Study the drawing (mm; zero at the part's minimum x, y, z) and answer. A direction names the side the tool comes from. Round coordinates to 2 decimals unless told otherwise and drop trailing zeros. Write each loop counter-clockwise with the first axis right and the second up, starting at its lowest first coordinate (ties: lowest second). Pieces come first, ordered by that corner, then holes. Notation, with made-up numbers: (59, -11.5) - (65, -11.5) arc R27 ccw to (65, 25.5) - close; hole circle Ø6 at (80, 0). An arc over 180 degrees is marked (long way). Return JSON: item names as keys, results as strings. Group by question number.
(1) Section A-A, the plane z = 55.5 is taken. Write down the section's boundary in (x, y), then the cut area to 3 significant figures.
(2) Which of the six approach directions +Z, -Z, +X, -X, +Y, -Y give full straight-line access (tool end or side, diameter ignored) to the marked faces 1 and 2?
(3) Section B-B, the plane x = 34 is taken. Write down the section's boundary in (y, z), then the cut area to 3 significant figures.
(4) Find the intervals of material crossed by line 1 along Y through (x, z) = (91, 95); line 2 along Z through (x, y) = (115, 172), in increasing order. Write a range as [from, to].
(5) This flat-tipped pin is pushed along its axis until it touches: pin 1 (4 mm diameter, centred on x = 173.5, y = 196, fed in from +Z). Where does it stop, or does it pass through?
(6) Determine the mould class of the marked faces 3, 4 and 5 for opening direction X: +X half, -X half, draft (parallel to the pull), parting line (faces both ways), or undercut.
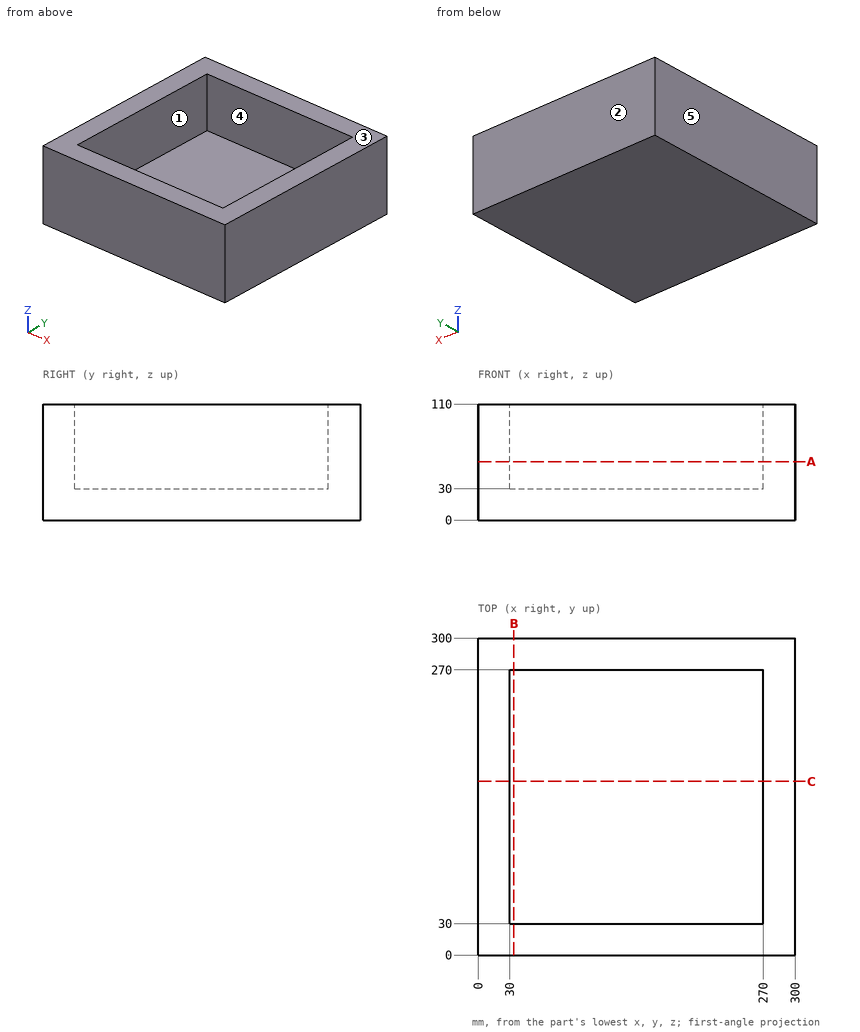
Working result:
{
 "1": {"outline": "(0, 0) - (300, 0) - (300, 300) - (0, 300) - close; hole (30, 30) - (270, 30) - (270, 270) - (30, 270) - close", "area": "32,400 mm^2"},
 "2": {"face 1": "+Z", "face 2": "+Z, -Z, +X, -X, +Y"},
 "3": {"outline": "(0, 0) - (300, 0) - (300, 110) - (270, 110) - (270, 30) - (30, 30) - (30, 110) - (0, 110) - close", "area": "13,800 mm^2"},
 "4": {"line 1": "y = [0, 30], [270, 300]", "line 2": "z = [0, 30]"},
 "5": {"pin 1": "stops at z = 30"},
 "6": {"face 3": "draft", "face 4": "undercut", "face 5": "-X half"}
}
